from build123d import *

# Parameters (mm, degrees)
BOSS_EXTRUDE1_DEPTH = 130
CUT_EXTRUDE1_DEPTH  = 10
CUT_EXTRUDE2_DEPTH  = 10


with BuildPart() as part:
    # Sketch1 → Boss-Extrude1 (new body)
    with BuildSketch(Plane(origin=(0, 0, 0), x_dir=(1, 0, 0), z_dir=(0, 1, 0))):
        Polygon((-95.340155061, -23.707512367), (-15.340155061, -23.707512367), (-15.340155061, 11.292487633), (-10.340155061, 11.292487633), (-10.340155061, -28.707512367), (-95.340155061, -28.707512367), align=None)
    extrude(amount=BOSS_EXTRUDE1_DEPTH)

    # Sketch2 → Cut-Extrude1 (cut)
    with BuildSketch(Plane.ZY.offset(15.340155061)):
        with BuildLine():
            Line((-11.292487633, 110), (20.707512367, 110))
            ThreePointArc((20.707512367, 110), (22.121725929, 109.414213562), (22.707512367, 108))
            Line((22.707512367, 108), (22.707512367, 102))
            ThreePointArc((22.707512367, 102), (22.121725929, 100.585786438), (20.707512367, 100))
            Line((20.707512367, 100), (-11.292487633, 100))
            Line((-11.292487633, 100), (-11.292487633, 110))
        make_face()
        with BuildLine():
            Line((-11.292487633, 30), (20.707512367, 30))
            ThreePointArc((20.707512367, 30), (22.121725929, 29.414213562), (22.707512367, 28))
            Line((22.707512367, 28), (22.707512367, 22))
            ThreePointArc((22.707512367, 22), (22.121725929, 20.585786438), (20.707512367, 20))
            Line((20.707512367, 20), (-11.292487633, 20))
            Line((-11.292487633, 20), (-11.292487633, 30))
        make_face()
    extrude(amount=-CUT_EXTRUDE1_DEPTH, mode=Mode.SUBTRACT)

    # Sketch3 → Cut-Extrude2 (cut)
    with BuildSketch(Plane(origin=(0, 0, 23.707512367), x_dir=(-1, 0, 0), z_dir=(0, 0, -1))):
        with BuildLine():
            Line((95.340155061, 100), (45.340155061, 100))
            ThreePointArc((45.340155061, 100), (43.925941499, 99.414213562), (43.340155061, 98))
            Line((43.340155061, 98), (43.340155061, 92))
            ThreePointArc((43.340155061, 92), (43.925941499, 90.585786438), (45.340155061, 90))
            Line((45.340155061, 90), (95.340155061, 90))
            Line((95.340155061, 90), (95.340155061, 100))
        make_face()
        with BuildLine():
            Line((95.340155061, 40), (45.340155061, 40))
            ThreePointArc((45.340155061, 40), (43.925941499, 39.414213562), (43.340155061, 38))
            Line((43.340155061, 38), (43.340155061, 32))
            ThreePointArc((43.340155061, 32), (43.925941499, 30.585786438), (45.340155061, 30))
            Line((45.340155061, 30), (95.340155061, 30))
            Line((95.340155061, 30), (95.340155061, 40))
        make_face()
    extrude(amount=-CUT_EXTRUDE2_DEPTH, mode=Mode.SUBTRACT)


solid = part.part
Source: CAD feature listing. Evaluate the final solid. Frame: model axes, mm. A direction names the side the tool comes from. Coordinates: 2 decimals unless noted, no trailing zeros. Write each loop counter-clockwise with the first axis right and the second up, starting at its lowest first coordinate (ties: lowest second). Pieces come first, ordered by that corner, then holes. Notation, with made-up numbers: M 44.25,61 L 81.25,61 A26 ccw 81.25,95 Z; hole C -28,66 d1. An arc over 180 degrees is marked long. Use a Markdown table: item, result.
1) Section D-D, the plane x = -28.5. Output: boundary loops of the cut face in (y, z), then the cut area to 3 significant figures.
Conclusion:
| item | result |
|---|---|
| outline | M 0,23.71 L 130,23.71 L 130,28.71 L 0,28.71 Z |
| area | 650 mm^2 |
2) Section C-C, the plane y = 73. Output: boundary loops of the cut face in (x, z), then the cut area to 3 significant figures.
Conclusion:
| item | result |
|---|---|
| outline | M -95.34,23.71 L -15.34,23.71 L -15.34,-11.29 L -10.34,-11.29 L -10.34,28.71 L -95.34,28.71 Z |
| area | 600 mm^2 |
3) Reachability of faces 5 (the flat face through (-13, 100, 5)), 6 (the flat face through (-71, 40, 26)), 7 (the flat face through (-56, 64, 23.708)) from +Z, -Z, +X, -X, +Y, -Y: full face, straight path, thin tool, end or side. Return the list, or none.
Conclusion:
| item | result |
|---|---|
| face 5 | -Z, +X, -X |
| face 6 | +Z, -Z, -X |
| face 7 | -Z, -X, +Y, -Y |
4) Ray query, L1, parallel to X at y = 97, z = 7.5; L2, parallel to Z at x = -29.5, y = 49. Return the intervals inside material, ascending.
Conclusion:
| item | result |
|---|---|
| L1 | x = -15.34 to -10.34 |
| L2 | z = 23.71 to 28.71 |
5) Mould query, pull axis Y, two halves, no side actions, for faces 1 (the flat face through (-15.34, 64, 6)), 2 (the flat face through (-37, 130, 25)), 3 (the flat face through (-43.34, 95, 26)), 4 (the flat face through (-37, 0, 25)). Classes: pulls with the +Y half, pulls with the -Y half, needs draft (parallel to the pull), parting line crosses it, or undercut.
Conclusion:
| item | result |
|---|---|
| face 1 | needs draft |
| face 2 | pulls with the +Y half |
| face 3 | undercut |
| face 4 | pulls with the -Y half |
6) Section A-A, the plane x = -80.5. Output: boundary loops of the cut face in (y, z), then the cut area to 3 significant figures.
Conclusion:
| item | result |
|---|---|
| outline | M 0,23.71 L 30,23.71 L 30,28.71 L 0,28.71 Z; M 40,23.71 L 90,23.71 L 90,28.71 L 40,28.71 Z; M 100,23.71 L 130,23.71 L 130,28.71 L 100,28.71 Z |
| area | 550 mm^2 |
7) Section B-B, the plane z = 18. Output: boundary loops of the cut face in (x, y).
Conclusion:
| item | result |
|---|---|
| outline | M -15.34,0 L -10.34,0 L -10.34,20 L -15.34,20 Z; M -15.34,30 L -10.34,30 L -10.34,100 L -15.34,100 Z; M -15.34,110 L -10.34,110 L -10.34,130 L -15.34,130 Z |
8) First-contact query: pin 1 Ø2.5 at (x, z) = (-63, 27) entering from -Y; pin 2 Ø1.5 at (y, z) = (77.5, 8) entering from -X; pin 3 Ø5.5 at (y, z) = (93.5, 26) entering from -X; pin 4 Ø2.5 at (x, y) = (-13, 25.5) entering from -Z. Flat tips, straight axial feed; report the tip coordinate or a pass-through.
Conclusion:
| item | result |
|---|---|
| pin 1 | stops at y = 0 |
| pin 2 | stops at x = -15.34 |
| pin 3 | stops at x = -43.78 |
| pin 4 | stops at z = 22.71 |
